Could you check a few things on this model? Use its own coordinates, in mm. A direction names the side the tool comes from. Coordinates: 2 decimals unless noted, no trailing zeros. Order: outer loops, then holes, each group sorted by start corner. A loop starts at its lowest first (then second) coordinate and runs counter-clockwise, first axis right, second up. Notation, with made-up numbers: M -32,22.5 L -18,22.5 A23 ccw -18,57.5 Z; hole C -16,41 d8. An arc over 180 degrees is marked long. Put each result on its own line as item: value. Start each with the question number.
```python
from build123d import *

# Parameters (mm, degrees)
SKETCH018_W           = 183.25
SKETCH018_H           = 152
SKETCH018_R           = 16.28
PAD006_DEPTH          = 8
SKETCH019_R           = 2.875
POCKET007_DEPTH       = 100
POCKET007_DEPTH_BACK  = 100
SKETCH020_R           = 5
POCKET008_DEPTH       = 3.1
SKETCH021_R           = 10
POCKET009_DEPTH       = 100
POCKET009_DEPTH_BACK  = 100
POLARPATTERN002_COUNT = 8


with BuildPart() as part:
    # Sketch018 → Pad006 (new body)
    with BuildSketch(Plane.XY):
        Rectangle(SKETCH018_W, SKETCH018_H)
        Circle(SKETCH018_R, mode=Mode.SUBTRACT)
        with BuildLine():
            ThreePointArc((-80.6875, 66.625), (-83.8125, 69.75), (-86.9375, 66.625))
            Line((-86.9375, 66.625), (-86.9375, -66.625))
            ThreePointArc((-86.9375, -66.625), (-83.8125, -69.75), (-80.6875, -66.625))
            Line((-80.6875, -66.625), (-80.6875, 66.625))
        make_face(mode=Mode.SUBTRACT)
        with BuildLine():
            ThreePointArc((86.9375, 66.625), (83.8125, 69.75), (80.6875, 66.625))
            Line((80.6875, 66.625), (80.6875, -66.625))
            ThreePointArc((80.6875, -66.625), (83.8125, -69.75), (86.9375, -66.625))
            Line((86.9375, -66.625), (86.9375, 66.625))
        make_face(mode=Mode.SUBTRACT)
    extrude(amount=PAD006_DEPTH)

    # Sketch019 (on Face15 of Pad006) → Pocket007 (cut, two sides)
    with BuildSketch(Plane.XY.offset(8)) as pocket007_sk:
        with Locations((-46.585079, 46.585079)):
            Circle(SKETCH019_R)
        with Locations((-46.585079, -46.585079)):
            Circle(SKETCH019_R)
        with Locations((46.585079, 46.585079)):
            Circle(SKETCH019_R)
        with Locations((46.585079, -46.585079)):
            Circle(SKETCH019_R)
        with Locations((-65.88125, 0)):
            Circle(SKETCH019_R)
        with Locations((0, -65.88125)):
            Circle(SKETCH019_R)
        with Locations((65.88125, 0)):
            Circle(SKETCH019_R)
        with Locations((0, 65.88125)):
            Circle(SKETCH019_R)
    extrude(amount=-POCKET007_DEPTH, mode=Mode.SUBTRACT)
    extrude(pocket007_sk.sketch, amount=POCKET007_DEPTH_BACK, mode=Mode.SUBTRACT)

    # Sketch020 (on Face4 of Pocket007) → Pocket008 (cut)
    with BuildSketch(Plane(origin=(0, 0, 0), x_dir=(1, 0, 0), z_dir=(0, 0, -1))):
        with Locations((-46.585079, 46.585079)):
            Circle(SKETCH020_R)
        with Locations((46.585079, 46.585079)):
            Circle(SKETCH020_R)
        with Locations((46.585079, -46.585079)):
            Circle(SKETCH020_R)
        with Locations((-46.585079, -46.585079)):
            Circle(SKETCH020_R)
    extrude(amount=-POCKET008_DEPTH, mode=Mode.SUBTRACT)

    # Sketch021 (on Face5 of Pocket008) → Pocket009 (cut, two sides)
    with BuildSketch(Plane.XY.offset(8)) as pocket009_sk:
        with Locations((-35, 0)):
            Circle(SKETCH021_R)
    pocket009 = extrude(amount=-POCKET009_DEPTH, mode=Mode.SUBTRACT) + extrude(pocket009_sk.sketch, amount=POCKET009_DEPTH_BACK, mode=Mode.SUBTRACT)

    # PolarPattern002: Pocket009 ×8 about axis
    polarpattern002_axis = Axis((0, 0, 8), (0, 0, 1))
    for i in range(1, POLARPATTERN002_COUNT):
        add(pocket009.rotate(polarpattern002_axis, i * 360 / POLARPATTERN002_COUNT), mode=Mode.SUBTRACT)


solid = part.part
```
Item 1: I need wall thicknesses on probe 1 along X at (y, z) = (-56, 1.5) (1 decimal); probe 2 along X at (y, z) = (24, 7) (1 decimal); probe 3 along X at (y, z) = (-39.5, 3.25) (1 decimal). Which ranges of each line are inside material? Lowest first, please.
Item 2: If we section it at A-A on y = -58.5: Write out the boundary of the cut face in (x, z) (1 decimal).
Item 3: For pin 1 Ø18 at (x, y) = (24.75, 24.75) entering from -Z; pin 2 Ø3 at (x, y) = (46.5, -48) entering from -Z, each with a flat end and sliding along its axis, tell me the tip position at first contact or that it passes through.
Item 4: If we section it at B-B on x = 0: Write out the boundary of the cut face in (y, z), then the cut area to 3 significant figures.
Item 5: If we mould it in two halves opening along X, with no side actions, what happens to faces 1 (the flat face through (19, 1, 8)), 2 (the flat face through (91.625, -1, 4)), 3 (the flat face through (-80.688, -1, 4))? For each: released by +X, released by -X, zero draft, split by the parting line, or undercut.
Item 6: For faces 4 (the flat face through (-86.938, 1, 4)), 5 (the flat face through (49, -44, 3.1)), 6 (the flat face through (-91.625, -1, 4)), which set-ups out of +Z, -Z, +X, -X, +Y, -Y let a thin tool reach every point of the face, with its end or its side?
Item 7: If we section it at D-D on y = -39.5: Write out the boundary of the cut face in (x, z) (1 decimal), then the cut area to 3 significant figures.
Item 8: If we section it at C-C on z = 1.75: State how many separate pieces and enclosed holes the cut face has, then the cut area to 3 significant figures.
Geometry check:
1. probe 1: x = -91.6 to -86.9, -80.7 to 80.7, 86.9 to 91.6
1. probe 2: x = -91.6 to -86.9, -80.7 to -34.7, -14.8 to 14.8, 34.7 to 80.7, 86.9 to 91.6
1. probe 3: x = -91.6 to -86.9, -80.7 to -8.9, 8.9 to 80.7, 86.9 to 91.6
2. outline: M -91.6,0 L -86.9,0 L -86.9,8 L -91.6,8 Z; M -80.7,0 L 80.7,0 L 80.7,8 L -80.7,8 Z; M 86.9,0 L 91.6,0 L 91.6,8 L 86.9,8 Z
3. pin 1: passes through
3. pin 2: stops at z = 3.1
4. outline: M -76,0 L -68.76,0 L -68.76,8 L -76,8 Z; M -63.01,0 L -45,0 L -45,8 L -63.01,8 Z; M -25,0 L -16.28,0 L -16.28,8 L -25,8 Z; M 16.28,0 L 25,0 L 25,8 L 16.28,8 Z; M 45,0 L 63.01,0 L 63.01,8 L 45,8 Z; M 68.76,0 L 76,0 L 76,8 L 68.76,8 Z
4. area: 544 mm²
5. face 1: zero draft
5. face 2: released by +X
5. face 3: undercut
6. face 4: +Z, -Z
6. face 5: -Z
6. face 6: +Z, -Z, -X, +Y, -Y
7. outline: M -91.6,0 L -86.9,0 L -86.9,8 L -91.6,8 Z; M -80.7,0 L -8.9,0 L -8.9,8 L -80.7,8 Z; M 8.9,0 L 80.7,0 L 80.7,8 L 8.9,8 Z; M 86.9,0 L 91.6,0 L 91.6,8 L 86.9,8 Z
7. area: 1,220 mm²
8. separate pieces: 1
8. enclosed holes: 19
8. area: 22,400 mm²
